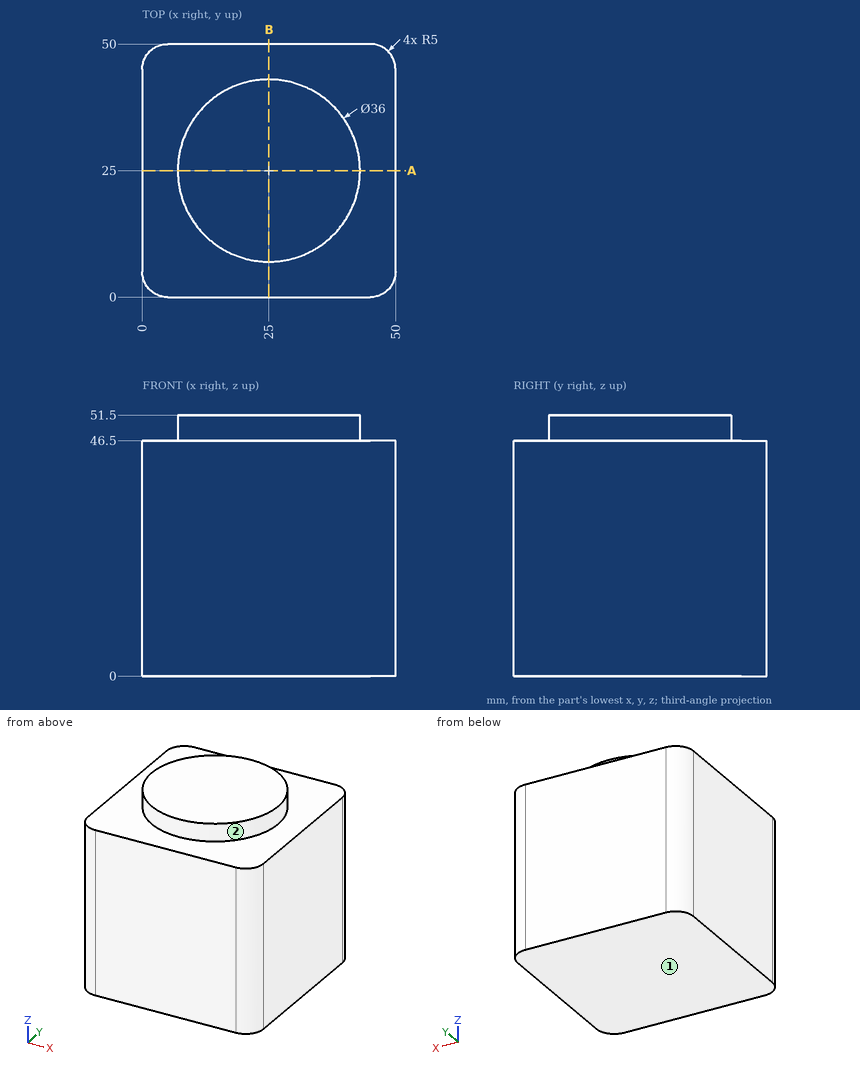
Design review of the part shown in the three views and the two pictorial views. Dimensions are in mm from the part's minimum x, y and z. A direction names the side the tool comes from. Coordinates: 2 decimals unless noted, no trailing zeros. Order: outer loops, then holes, each group sorted by start corner. A loop starts at its lowest first (then second) coordinate and runs counter-clockwise, first axis right, second up.
Item 1: Take a section at A-A, the plane y = 25. Write out the cut boundary in (x, z).
Item 2: For line 1 (Z direction, x = 41.5, y = 44); line 2 (Y direction, x = 45.5, z = 32); line 3 (Y direction, x = 48, z = 24), list the stretches that pass through material, from the lowest coordinate up.
Item 3: For the marked faces 1 and 2, list the 3-axis set-ups (+Z, -Z, +X, -X, +Y, -Y) from which the entire face can be reached by the end or side of a thin tool; tool diameter is ignored.
The answers:
1. outline: (0, 0) - (50, 0) - (50, 46.5) - (43, 46.5) - (43, 51.5) - (7, 51.5) - (7, 46.5) - (0, 46.5) - close
2. line 1: z = 0 to 46.5
2. line 2: y = 0.03 to 49.97
2. line 3: y = 1 to 49
3. face 1: -Z, +X, -X, +Y, -Y
3. face 2: +Z
